Can you work these out from the model? Positions are in its coordinate system, mm. A direction names the side the tool comes from. Give positions to 0.01 mm unless a question says otherwise; leave off trailing zeros. Loops run counter-clockwise (first coordinate to the right, second up) from the corner with the lowest first, then second, coordinate; pieces in that order, holes last. Notation, with made-up numbers: M 6,60 L 40,60 A20 cw 40,83 Z; hole C -18,47.5 d7. An arc over 180 degrees is marked long. Answer as a JSON object with one key per item and string values.
Solid Edge part; units mm, degrees
sketch "Sketch1" plane through (0, 0, 0) normal (0, 0, 1) x (1, 0, 0)
  line L0 (2, 0) -> (2, 6)
  line L1 (0, 6) -> (2, 6)
  line L2 (0, 0) -> (0, 6)
  line L3 (0, 0) -> (0, -4)
  line L4 (0, -4) -> (3.5, -4)
  line L5 (3.5, -4) -> (3.5, 0)
  line L6 (3.5, 0) -> (2, 0)
revolve "RevolvedProtrusion1" add sketch "Sketch1" angle 360 about axis through (0, 0, 0) along (0, 1, 0)
sketch "Sketch2" plane through (0, 0, 0) normal (1, 0, 0) x (0, 1, 0)
  line L0 (-4, 2.2215) -> (-2, 2.2215)
  line L1 (-0.7174, 0) -> (-2, 2.2215)
  line L2 (-4, 0) -> (-0.7174, 0)
  line L3 (-4, 0) -> (-4, 2.2215)
revolve "RevolvedCutout1" cut sketch "Sketch2" angle 360 about axis through (0, -4.5, 0) along (0, 1, 0)
sketch "Sketch3" plane through (0, -4, 0) normal (0, -1, 0) x (0, 0, 1)
  circle A0 centre (0, 0) radius 2.2215
  line L0 (-1.5, -0.866) -> (0, -1.7321)
  line L1 (0, -1.7321) -> (1.5, -0.866)
  line L2 (1.5, -0.866) -> (1.5, 0.866)
  line L3 (1.5, 0.866) -> (0, 1.7321)
  line L4 (0, 1.7321) -> (-1.5, 0.866)
  line L5 (-1.5, 0.866) -> (-1.5, -0.866)
extrude "Protrusion1" add sketch "Sketch3" against normal up to next
sketch "Sketch4" plane through (0, 0, 0) normal (0, 0, 1) x (1, 0, 0)
  line L0 (-1.7321, -4) -> (0, -4)
  line L1 (0, -4) -> (0, -3.5359)
  line L2 (0, -3.5359) -> (-1.7321, -4)
revolve "RevolvedCutout2" cut sketch "Sketch4" angle 360 about axis through (0, -4.5, 0) along (0, 1, 0)
fillet "Round1" radius 0.2 1 edges at (0, 0, -2)
fillet "Round2" radius 0.35 1 edges at (0, -4, -3.5)
chamfer "倒斜角_2" distance 0.2667 angle 45 1 edges at (0, 6, -2)
cosmetic_thread "螺纹_3" thread depth 4.8
1) Will this pin go through, and if not, where does the flat tip stop? pin 1 Ø3 at (y, z) = (3.5, 0) entering from -X.
Answer list:
{"pin 1": "x = -2"}
2) Please list where these lines run through material, in increasing order: line 1 along Y through (x, z) = (1.5, 0); line 2 along Y through (x, z) = (-2.75, 1.5); line 3 along Z through (x, y) = (0.25, -1.75). Write a range as from..to.
Answer list:
{"line 1": "-1.58..6", "line 2": "-4..0", "line 3": "-3.49..-1.5, 1.5..3.49"}
3) For faces 1 (the flat face through (0, -3, -1.5)), 2 (the flat face through (-2, 0, 2)), 3 (the cylindrical face through (3.233, -1.799, 1.341)), which set-ups out of +Z, -Z, +X, -X, +Y, -Y let a thin tool reach every point of the face, with its end or its side?
Answer list:
{"face 1": "-Y", "face 2": "+Y", "face 3": "+Y, -Y"}
4) If we mould it in two halves opening along X, with no side actions, what happens to faces 4 (the cylindrical face through (0, 3, 2)), 5 (the flat face through (1.305, -2.809, 0.739)), 6 (the flat face through (1.4, -4, 1.4))? For each: +X half, -X half, draft (parallel to the pull), parting line (faces both ways), or undercut.
Answer list:
{"face 4": "parting line", "face 5": "undercut", "face 6": "draft"}
5) Suppose I cut it at A-A, the plane y = 4.25. Write out the boundary of the cut face in (x, z), and give its area (3 significant figures).
Answer list:
{"outline": "C 0,0 d4", "area": "12.6 mm^2"}
